Read the model definition and answer for the solid it produces. Units are mm, in the model's axes. A direction names the side the tool comes from. Give positions to 0.01 mm unless a question says otherwise; leave off trailing zeros. Order: outer loops, then holes, each group sorted by start corner. A loop starts at its lowest first (then second) coordinate and runs counter-clockwise, first axis right, second up. Notation, with made-up numbers: (60.5, 86) -> (95.5, 86) arc R28 ccw to (95.5, 124) -> close; hole circle Ø9 at (51, -33.5). An arc over 180 degrees is marked (long way). Answer as CSV lines item,"result". Start each with the question number.
1) Find section B-B (x = 34.5). Determine the outline of the cut face in (y, z).
2) Find section A-A (y = 21). Determine the outline of the cut face in (x, z).
3) Find section D-D (z = -1.75). Determine the outline of the cut face in (x, y).
4) The mould has two halves that part along Y. Classify faces 1 (the face through (49.324, 1.159, 0.789)), 2 (the face through (48, 16, 7.16)), 3 (the face through (27, 6.2, -3)), 4 (the face through (4.884, 2.487, 0.789)): +Y half, -Y half, draft (parallel to the pull), parting line (faces both ways), or undercut.
5) For faces 5 (the face through (29.995, -0.608, 12.052)), 6 (the face through (48, 23.2, 4)), 7 (the face through (22.337, 4, -2)), determine the directions among +Z, -Z, +X, -X, +Y, -Y from which every point of the face is accessible in a straight line to the end or side of a thin tool.
6) Flat-ended cylindrical pins translate along their axes: pin 1 Ø4 at (x, y) = (6, 34) entering from -Z; pin 2 Ø2 at (x, z) = (17, -0.5) entering from +Y; pin 3 Ø1.4 at (y, z) = (15.5, 4.5) entering from +X; pin 4 Ø5.5 at (x, y) = (4.064, 4.064) entering from +Z. Find the tip coordinate at first contact, or state that the pin passes through.
7) Find section C-C (z = 13.5). Determine the outline of the cut face in (x, y), and give its area (3 significant figures).
8) Straight lines are drawn through the part: L1, parallel to Z at x = 20, y = 3; L2, parallel to X at y = 20.5, z = 3.5; L3, parallel to X at y = 26, z = 8. For each, find the intervals that lie inside material, in ascending order. Write a range as from..to.
```python
from build123d import *

# Parameters (mm, degrees)
SKETCH_R     = 1.778
PAD_DEPTH    = 1.6
SKETCH001_W  = 2.16
SKETCH001_H  = 20.66
PAD001_DEPTH = 10.88
PAD002_DEPTH = 4.48
SKETCH003_W  = 8.8
SKETCH003_H  = 7.28
PAD003_DEPTH = 3.1
FILLET_R     = 1.5
SKETCH004_W  = 17.8
SKETCH004_H  = 28.4
PAD004_DEPTH = 1.1
SKETCH005_W  = 9
SKETCH005_H  = 6.8
PAD005_DEPTH = 3.1
FILLET001_R  = 1.5
SKETCH006_W  = 7.8
SKETCH006_H  = 15
PAD006_DEPTH = 5.56
SKETCH007_W  = 4.3
SKETCH007_H  = 8.64
PAD007_DEPTH = 4.6
SKETCH008_W  = 2
SKETCH008_H  = 2
PAD008_DEPTH = 3.9
SKETCH009_W  = 5.9
SKETCH009_H  = 7.9
PAD009_DEPTH = 4.56
SKETCH010_W  = 10
SKETCH010_H  = 9.7
PAD010_DEPTH = 2.78
SKETCH011_W  = 17.8
SKETCH011_H  = 19
PAD011_DEPTH = 1.3


with BuildPart() as part:
    # Sketch → Pad (new body)
    with BuildSketch(Plane.XY):
        with BuildLine():
            Line((4.064, 0), (46.482, 0))
            ThreePointArc((46.482, 0), (49.355682, 1.190318), (50.546, 4.064))
            Line((50.546, 4.064), (50.546, 39.878))
            ThreePointArc((50.546, 39.878), (49.355682, 42.751682), (46.482, 43.942))
            Line((46.482, 43.942), (4.064, 43.942))
            ThreePointArc((4.064, 43.942), (1.190318, 42.751682), (0, 39.878))
            Line((0, 39.878), (0, 4.064))
            ThreePointArc((0, 4.064), (1.190318, 1.190318), (4.064, 0))
        make_face()
        with Locations((4.064, 39.878)):
            Circle(SKETCH_R, mode=Mode.SUBTRACT)
        with Locations((46.482, 39.878)):
            Circle(SKETCH_R, mode=Mode.SUBTRACT)
        with Locations((46.482, 4.064)):
            Circle(SKETCH_R, mode=Mode.SUBTRACT)
        with Locations((4.064, 4.064)):
            Circle(SKETCH_R, mode=Mode.SUBTRACT)
    extrude(amount=PAD_DEPTH)

    # Sketch001 (on Face14 of Pad) → Pad001 (join)
    with BuildSketch(Plane.XY.offset(1.6)):
        with Locations((15.18, 17.21)):
            Rectangle(SKETCH001_W, SKETCH001_H)
        with Locations((38.366, 17.21)):
            Rectangle(SKETCH001_W, SKETCH001_H)
    extrude(amount=PAD001_DEPTH)

    # Sketch002 (on Face23 of Pad001) → Pad002 (join)
    with BuildSketch(Plane.XY.offset(12.48)):
        with BuildLine():
            Line((14.1, 6.88), (14.1, 32.15))
            ThreePointArc((16.2, 34.25), (14.715076, 33.634924), (14.1, 32.15))
            Line((16.2, 34.25), (37.346, 34.25))
            ThreePointArc((39.446, 32.15), (38.830924, 33.634924), (37.346, 34.25))
            Line((39.446, 0), (39.446, 32.15))
            Line((15.9, 0), (39.446, 0))
            Line((15.9, 5.28), (15.9, 0))
            ThreePointArc((15.9, 5.28), (15.431371, 6.411371), (14.3, 6.88))
            Line((14.1, 6.88), (14.3, 6.88))
        make_face()
    extrude(amount=PAD002_DEPTH)

    # Sketch003 (on Face24 of Pad002) → Pad003 (join)
    with BuildSketch(Plane(origin=(0, 0, 12.48), x_dir=(1, 0, 0), z_dir=(0, 0, -1))):
        with Locations((26.046, -2.44)):
            Rectangle(SKETCH003_W, SKETCH003_H)
    extrude(amount=PAD003_DEPTH)

    # Fillet
    fillet_edges = [part.edges().sort_by_distance(p)[0] for p in [
        (21.646, -0.6, 12.48),
        (30.446, -0.6, 12.48),
        (30.446, 2.44, 9.38),
        (21.646, 2.44, 9.38),
    ]]
    fillet(fillet_edges, radius=FILLET_R)

    # Sketch004 (on Face43 of Fillet) → Pad004 (join)
    with BuildSketch(Plane(origin=(0, 0, 0), x_dir=(1, 0, 0), z_dir=(0, 0, -1))):
        with Locations((26.837, -14.2)):
            Rectangle(SKETCH004_W, SKETCH004_H)
    extrude(amount=PAD004_DEPTH)

    # Sketch005 (on Face48 of Pad004) → Pad005 (join)
    with BuildSketch(Plane(origin=(0, 0, -1.1), x_dir=(1, 0, 0), z_dir=(0, 0, -1))):
        with Locations((26.837, -2.8)):
            Rectangle(SKETCH005_W, SKETCH005_H)
    extrude(amount=PAD005_DEPTH)

    # Fillet001
    fillet001_edges = [part.edges().sort_by_distance(p)[0] for p in [
        (31.337, -0.3, -1.1),
        (22.337, -0.3, -1.1),
        (31.337, 2.8, -4.2),
        (22.337, 2.8, -4.2),
    ]]
    fillet(fillet001_edges, radius=FILLET001_R)

    # Sketch006 (on Face19 of Fillet001) → Pad006 (join)
    with BuildSketch(Plane.XY.offset(1.6)):
        with Locations((47.846, 15.7)):
            Rectangle(SKETCH006_W, SKETCH006_H)
    extrude(amount=PAD006_DEPTH)

    # Sketch007 (on Face19 of Pad006) → Pad007 (join)
    with BuildSketch(Plane.XY.offset(1.6)):
        with Locations((47.996, 30.522)):
            Rectangle(SKETCH007_W, SKETCH007_H)
    extrude(amount=PAD007_DEPTH)

    # Sketch008 (on Face43 of Pad007) → Pad008 (join)
    with BuildSketch(Plane.YZ.offset(50.146)):
        with Locations((31.642, 4.14)):
            Rectangle(SKETCH008_W, SKETCH008_H)
        with Locations((29.402, 4.14)):
            Rectangle(SKETCH008_W, SKETCH008_H)
    extrude(amount=PAD008_DEPTH)

    # Sketch009 (on Face19 of Pad008) → Pad009 (join)
    with BuildSketch(Plane.XY.offset(1.6)):
        with Locations((5.25, 14.45)):
            Rectangle(SKETCH009_W, SKETCH009_H)
    extrude(amount=PAD009_DEPTH)

    # Sketch010 (on Face19 of Pad009) → Pad010 (join)
    with BuildSketch(Plane.XY.offset(1.6)):
        with Locations((6.6, 28.392)):
            Rectangle(SKETCH010_W, SKETCH010_H)
    extrude(amount=PAD010_DEPTH)

    # Sketch011 (on Face7 of Pad010) → Pad011 (join)
    with BuildSketch(Plane(origin=(0, 0, -1.1), x_dir=(1, 0, 0), z_dir=(0, 0, -1))):
        with Locations((26.837, -18.9)):
            Rectangle(SKETCH011_W, SKETCH011_H)
    extrude(amount=PAD011_DEPTH)


solid = part.part
```
Findings below:
1,outline,"(0, -1.1) -> (9.4, -1.1) -> (9.4, -2.4) -> (28.4, -2.4) -> (28.4, 0) -> (43.94, 0) -> (43.94, 1.6) -> (0, 1.6) -> close; (0, 12.48) -> (34.25, 12.48) -> (34.25, 16.96) -> (0, 16.96) -> close"
2,outline,"(0, 0) -> (17.94, 0) -> (17.94, -2.4) -> (35.74, -2.4) -> (35.74, 0) -> (50.55, 0) -> (50.55, 1.6) -> (51.75, 1.6) -> (51.75, 7.16) -> (43.95, 7.16) -> (43.95, 1.6) -> (39.45, 1.6) -> (39.45, 16.96) -> (14.1, 16.96) -> (14.1, 1.6) -> (0, 1.6) -> close; hole (16.26, 1.6) -> (37.29, 1.6) -> (37.29, 12.48) -> (16.26, 12.48) -> close"
3,outline,"(17.94, 9.4) -> (35.74, 9.4) -> (35.74, 28.4) -> (17.94, 28.4) -> close; (22.34, 0) -> (22.6, 0) -> (22.6, -0.6) -> (31.07, -0.6) -> (31.07, 0) -> (31.34, 0) -> (31.34, 6.2) -> (22.34, 6.2) -> close"
4,face 1,"-Y half"
4,face 2,"draft"
4,face 3,"undercut"
4,face 4,"undercut"
5,face 5,"+Z, +X, -Y"
5,face 6,"+Z, +X"
5,face 7,"-Z, -X, -Y"
6,pin 1,"z = 0"
6,pin 2,"y = 43.94"
6,pin 3,"x = 51.75"
6,pin 4,"z = 1.6"
7,outline,"(14.1, 6.88) -> (14.3, 6.88) arc R1.6 cw to (15.9, 5.28) -> (15.9, 0) -> (39.45, 0) -> (39.45, 32.15) arc R2.1 ccw to (37.35, 34.25) -> (16.2, 34.25) arc R2.1 ccw to (14.1, 32.15) -> close"
7,area,"854 mm²"
8,L1,"-1.1..1.6, 12.48..16.96"
8,L2,"14.1..16.26, 37.29..39.45, 43.95..51.75"
8,L3,"14.1..16.26, 37.29..39.45"
